Here's how the part is built. I have some questions about the finished solid (model axes, mm). A direction names the side the tool comes from. Round coordinates to 2 decimals unless told otherwise and drop trailing zeros. Write each loop counter-clockwise with the first axis right and the second up, starting at its lowest first coordinate (ties: lowest second). Pieces come first, ordered by that corner, then holes. Notation, with made-up numbers: (22.5, -18.5) - (26.5, -18.5) arc R13 cw to (26.5, -5.5) - close; hole circle Ø11 at (-2.75, 52.25). An arc over 180 degrees is marked (long way). One line per item, written item: value. Start each with the question number.
Item 1: If I drill on line 1 (Y direction, x = 14.75, z = 36); line 2 (Z direction, x = 23, y = -12); line 3 (Y direction, x = 15.75, z = 38), over which ranges is the centre line in solid material (lowest first)?
Item 2: Imagine slicing it at C-C, the plane z = -3. Please give me the cut outline in (x, y).
Item 3: Imagine slicing it at B-B, the plane x = 18.25. Count the separate pieces of the cut face and the enclosed holes in it, then the cut area to 3 significant figures.
Item 4: For faces 5 (the face through (10, -12, 36)), 6 (the face through (21, -12, -3)), 7 (the face through (18, 0, 11)), which set-ups out of +Z, -Z, +X, -X, +Y, -Y let a thin tool reach every point of the face, with its end or its side?
Item 5: Imagine slicing it at A-A, the plane z = 36. Please give me the cut outline in (x, y).
Item 6: For P1, Ø1, axis at x = 11, y = -21, coming from the -Z side; P2, Ø1.5, axis at y = -13, z = 20.5, coming from the -X side; P3, Ø3.5, axis at y = -4, z = -3, coming from the +X side; P4, Ø7, axis at y = -11, z = 36, coming from the -X side, each with a flat end and sliding along its axis, tell me the tip position at first contact or that it passes through.
Item 7: Imagine slicing it at D-D, the plane x = 8. Please give me the cut outline in (y, z), then the cut area to 3 significant figures.
Item 8: Thinking about a two-plate mould opening in Z: for faces 1 (the face through (6, -12, -4)), 2 (the face through (17.741, -2.108, 33.936)), 3 (the face through (12, -12, 40.994)), 4 (the face through (17.74, -11.83, -7.62)), which applies, released by +Z, released by -Z, zero draft, split by the parting line, or undercut?
```python
from build123d import *

# Parameters (mm, degrees)
CYLINDER014_R     = 2.3
CYLINDER014_DEPTH = 20
CYLINDER015_R     = 2.3
CYLINDER015_DEPTH = 20
CYLINDER004_R     = 2.8
CYLINDER004_DEPTH = 60
CYLINDER005_R     = 2.8
CYLINDER005_DEPTH = 60
CYLINDER006_R     = 2.8
CYLINDER006_DEPTH = 60
CYLINDER007_R     = 2.8
CYLINDER007_DEPTH = 60
PAD003_DEPTH      = 24


with BuildPart() as obj1:
    # Cylinder014 → Cylinder014 (new body)
    with BuildSketch(Plane(origin=(41, -12, -3), x_dir=(0, 0, 1), z_dir=(-1, 0, 0))):
        Circle(CYLINDER014_R)
    extrude(amount=CYLINDER014_DEPTH)


with BuildPart() as obj2:
    # Cylinder015 → Cylinder015 (new body)
    with BuildSketch(Plane(origin=(41, -12, 36), x_dir=(0, 0, 1), z_dir=(-1, 0, 0))):
        Circle(CYLINDER015_R)
    extrude(amount=CYLINDER015_DEPTH)


with BuildPart() as o003:
    # Cylinder004 → Cylinder004 (new body)
    with BuildSketch(Plane(origin=(41, -4, 36), x_dir=(0, 0, 1), z_dir=(-1, 0, 0))):
        Circle(CYLINDER004_R)
    extrude(amount=CYLINDER004_DEPTH)


with BuildPart() as u003:
    # Cylinder005 → Cylinder005 (new body)
    with BuildSketch(Plane(origin=(41, -20, -3), x_dir=(0, 0, 1), z_dir=(-1, 0, 0))):
        Circle(CYLINDER005_R)
    extrude(amount=CYLINDER005_DEPTH)


with BuildPart() as u004:
    # Cylinder006 → Cylinder006 (new body)
    with BuildSketch(Plane(origin=(41, -4, -3), x_dir=(0, 0, 1), z_dir=(-1, 0, 0))):
        Circle(CYLINDER006_R)
    extrude(amount=CYLINDER006_DEPTH)


with BuildPart() as o004:
    # Cylinder007 → Cylinder007 (new body)
    with BuildSketch(Plane(origin=(41, -20, 36), x_dir=(0, 0, 1), z_dir=(-1, 0, 0))):
        Circle(CYLINDER007_R)
    extrude(amount=CYLINDER007_DEPTH)


with BuildPart() as cut020:
    # Sketch003 → Pad003 (new body)
    with BuildSketch(Plane.XZ):
        with BuildLine():
            ThreePointArc((6, 0.701169), (11.288851, 3.875794), (10.727222, 10.018656))
            add(Edge.make_bspline(
                [(10.727222, 10.018656), (21.113006, 10.736894), (20.761279, 21.365217), (20.409553, 31.993539), (10, 31.993539)],
                knots=[3.209183, 3.209183, 3.209183, 4.746184, 4.746184, 6.283185, 6.283185, 6.283185], degree=2, weights=[1, 0.718954, 1, 0.718954, 1]))
            Line((10, 31.993539), (10, 40.993539))
            Line((10, 40.993539), (14, 40.993539))
            Line((14, 40.993539), (25.267428, 40.007767))
            Line((25.267428, 40.007767), (25.267428, -6.963104))
            Line((25.267428, -6.963104), (10, -8.298831))
            Line((10, -8.298831), (6, -8.298831))
            Line((6, -8.298831), (6, 0.701169))
        make_face()
    extrude(amount=PAD003_DEPTH)

    # Cut015: cut O004
    add(o004.part, mode=Mode.SUBTRACT)

    # Cut016: cut U004
    add(u004.part, mode=Mode.SUBTRACT)

    # Cut017: cut U003
    add(u003.part, mode=Mode.SUBTRACT)

    # Cut018: cut O003
    add(o003.part, mode=Mode.SUBTRACT)

    # Cut019: cut obj2
    add(obj2.part, mode=Mode.SUBTRACT)

    # Cut020: cut obj1
    add(obj1.part, mode=Mode.SUBTRACT)


solid = cut020.part
```
Values follow:
1. line 1: y = -24 to -22.8, -17.2 to -6.8, -1.2 to 0
1. line 2: z = -7.16 to -5.3, -0.7 to 33.7, 38.3 to 40.21
1. line 3: y = -24 to -21.96, -18.04 to -5.96, -2.04 to 0
2. outline: (6, -24) - (25.27, -24) - (25.27, -22.8) - (6, -22.8) - close; (6, -17.2) - (25.27, -17.2) - (25.27, -14.3) - (21, -14.3) - (21, -9.7) - (25.27, -9.7) - (25.27, -6.8) - (6, -6.8) - close; (6, -1.2) - (25.27, -1.2) - (25.27, 0) - (6, 0) - close
3. separate pieces: 2
3. enclosed holes: 4
3. area: 719 mm^2
4. face 5: +Z, -X, +Y, -Y
4. face 6: +X
4. face 7: +Z, -Z, +X, -X, +Y
5. outline: (10, -24) - (25.27, -24) - (25.27, -22.8) - (10, -22.8) - close; (10, -17.2) - (25.27, -17.2) - (25.27, -14.3) - (21, -14.3) - (21, -9.7) - (25.27, -9.7) - (25.27, -6.8) - (10, -6.8) - close; (10, -1.2) - (25.27, -1.2) - (25.27, 0) - (10, 0) - close
6. P1: stops at z = -8.26
6. P2: stops at x = 20.7
6. P3: passes through
6. P4: stops at x = 10
7. outline: (-24, -8.3) - (0, -8.3) - (0, 1.01) - (-24, 1.01) - close; hole circle Ø5.6 at (-20, -3); hole circle Ø5.6 at (-4, -3)
7. area: 174 mm^2
8. face 1: zero draft
8. face 2: undercut
8. face 3: released by +Z
8. face 4: released by -Z
